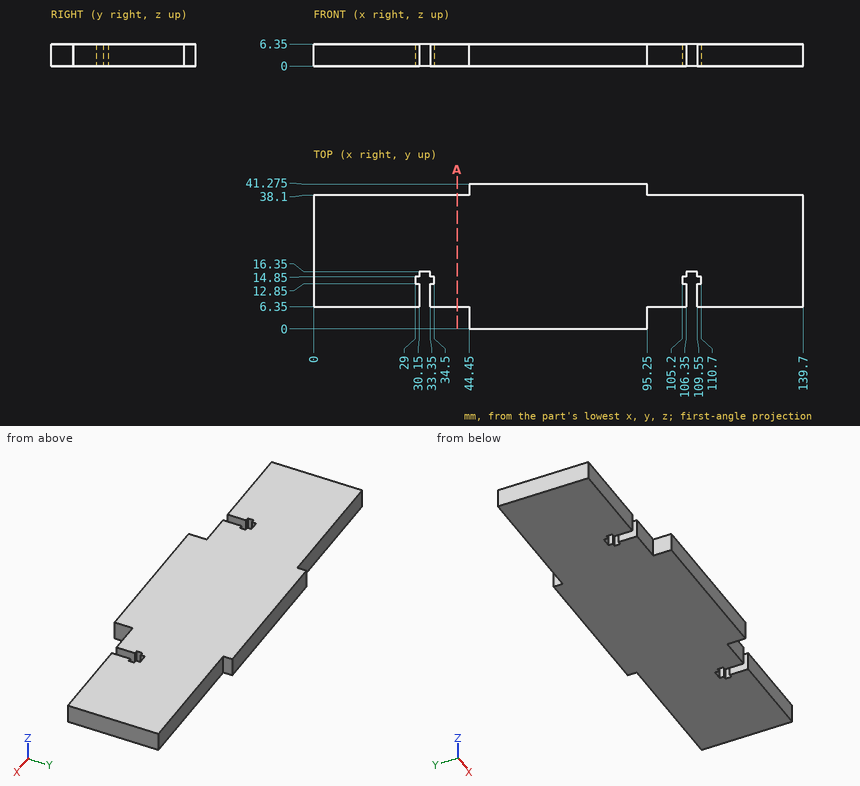
Part print with two shaded views. Sizes in mm from the minimum x, y, z corner. Coordinates: 2 decimals unless noted, no trailing zeros. Order: outer loops, then holes, each group sorted by start corner. A loop starts at its lowest first (then second) coordinate and runs counter-clockwise, first axis right, second up. Notation, with made-up numbers: M 8,82 L 49,82 A31 cw 49,111 Z; hole C -38.5,-36 d8. An arc over 180 degrees is marked long. One line per question, with ' | ' between items. Start each with the question number.
1. Cut at A-A (x = 41). Write the cut outline in (y, z).
2. Flat gauge pins, fed straight in: P1, Ø0.6, axis at x = 30, z = 3, coming from the +Y side; P2, Ø3, axis at x = 20.5, z = 1.5, coming from the -Y side; P3, Ø1.9, axis at y = 2, z = 3.5, coming from the -X side. Where does each tip first touch, or does it go through?
3. Wall check: line 1 along X through (y, z) = (8, 5); line 2 along Y through (x, z) = (96, 4.25); line 3 along X through (y, z) = (39, 4.5). Give the ranges that are in metal, low to high. Write a range as [from, to].
The answers:
1) outline: M 6.35,0 L 38.1,0 L 38.1,6.35 L 6.35,6.35 Z
2) P1: stops at y = 38.1 | P2: stops at y = 6.35 | P3: stops at x = 44.45
3) line 1: x = [0, 30.15], [33.35, 106.35], [109.55, 139.7] | line 2: y = [6.35, 38.1] | line 3: x = [44.45, 95.25]
